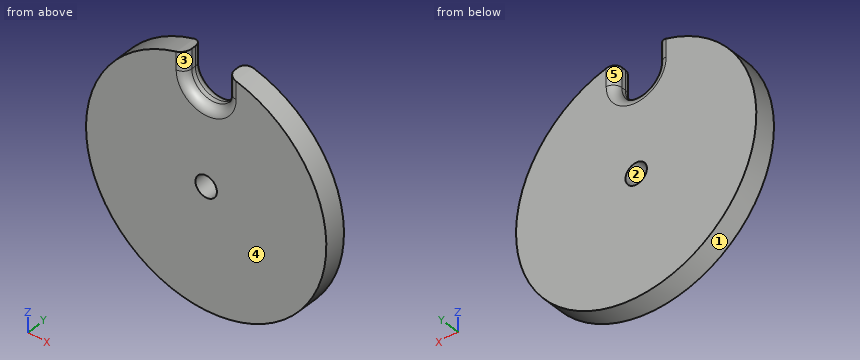
from build123d import *

# Parameters (mm, degrees)
SKETCH2_R                  = 35.56
BOSS_EXTRUDE1_DEPTH        = 6.35
SHOCK_CORD_HOLE_DEPTH      = 1
SHOCK_CORD_HOLE_DEPTH_BACK = 7.35
FILLET1_R                  = 2.54
SKETCH18_R                 = 3.175
CUT_EXTRUDE1_DEPTH         = 7.3500001


with BuildPart() as part:
    # Sketch2 → Boss-Extrude1 (new body)
    with BuildSketch(Plane(origin=(0, 0, 0), x_dir=(1, 0, 0), z_dir=(0, 1, 0))):
        Circle(SKETCH2_R)
    extrude(amount=BOSS_EXTRUDE1_DEPTH)

    # Sketch4 → Shock Cord hole (cut, two sides)
    with BuildSketch(Plane(origin=(0, 6.35, 0), x_dir=(1, 0, 0), z_dir=(0, 1, 0))) as shock_cord_hole_sk:
        with BuildLine():
            Line((6.35, -209.104630755), (6.35, -34.988442377))
            Line((6.35, -34.988442377), (6.35, -29.21))
            ThreePointArc((6.35, -29.21), (0, -22.86), (-6.35, -29.21))
            Line((-6.35, -29.21), (-6.35, -34.988442377))
            Line((-6.35, -34.988442377), (-6.35, -209.104630755))
            Line((-6.35, -209.104630755), (-6.35, -557.33700751))
            Line((-6.35, -557.33700751), (6.35, -557.33700751))
            Line((6.35, -557.33700751), (6.35, -209.104630755))
        make_face()
    extrude(amount=SHOCK_CORD_HOLE_DEPTH, mode=Mode.SUBTRACT)
    extrude(shock_cord_hole_sk.sketch, amount=-SHOCK_CORD_HOLE_DEPTH_BACK, mode=Mode.SUBTRACT)

    # Fillet1
    fillet1_edges = [part.edges().sort_by_distance(p)[0] for p in [
        (-6.35, 6.35, 32.099221189),
        (0, 6.35, 22.86),
        (6.35, 6.35, 32.099221189),
        (6.35, 0, 32.099221189),
        (0, 0, 22.86),
        (-6.35, 0, 32.099221189),
    ]]
    fillet(fillet1_edges, radius=FILLET1_R)

    # Sketch18 → Cut-Extrude1 (cut, through all)
    with BuildSketch(Plane.XZ):
        Circle(SKETCH18_R)
    extrude(amount=-CUT_EXTRUDE1_DEPTH, mode=Mode.SUBTRACT)


solid = part.part
Input: part model. Units: mm. Frame: model coordinates. Face numbers are marked on the shaded views. A direction names the side the tool comes from. Round coordinates to 2 decimals unless told otherwise and drop trailing zeros. Order: outer loops, then holes, each group sorted by start corner. A loop starts at its lowest first (then second) coordinate and runs counter-clockwise, first axis right, second up. Notation, with made-up numbers: (79.5, 56) - (99.5, 56) arc R15 ccw to (99.5, 63) - close; hole circle Ø10 at (79.5, 16). An arc over 180 degrees is marked (long way). Use a Markdown table: item, result.
1. Material intervals for probe 1 along Z at (x, y) = (0, 3) (3 decimals); probe 2 along X at (y, z) = (2.25, 0.5); probe 3 along X at (y, z) = (2.5, -2.5), sorted ascending.
Evaluation:
| item | result |
|---|---|
| probe 1 | -35.56 to -3.175, 3.175 to 22.86 |
| probe 2 | -35.56 to -3.14, 3.14 to 35.56 |
| probe 3 | -35.47 to -1.96, 1.96 to 35.47 |
2. Section A-A on x = 0. Return the cut outline in (y, z) (3 decimals), then the cut area to 3 significant figures.
Evaluation:
| item | result |
|---|---|
| outline | (0, -35.56) - (6.35, -35.56) - (6.35, -3.175) - (0, -3.175) - close; (0, 3.175) - (6.35, 3.175) - (6.35, 20.32) arc R2.54 ccw to (3.81, 22.86) - (2.54, 22.86) arc R2.54 ccw to (0, 20.32) - close |
| area | 328 mm^2 |
3. Mould query, pull axis Z, two halves, no side actions, for the marked faces 1, 2 and 3. Classes: +Z half, -Z half, draft (parallel to the pull), parting line (faces both ways), or undercut.
Evaluation:
| item | result |
|---|---|
| face 1 | parting line |
| face 2 | undercut |
| face 3 | draft |
4. Section D-D on z = -26.5. Return the cut outline in (x, y), then the cut area to 3 significant figures.
Evaluation:
| item | result |
|---|---|
| outline | (-23.71, 0) - (23.71, 0) - (23.71, 6.35) - (-23.71, 6.35) - close |
| area | 301 mm^2 |
5. Section C-C on y = 1.5. Return the cut outline in (x, z) (3 decimals).
Evaluation:
| item | result |
|---|---|
| outline | (-6.573, 29.21) - (-6.573, 34.947) arc R35.56 ccw (long way) to (6.573, 34.947) - (6.573, 29.21) arc R6.573 cw to start; hole circle Ø6.35 at (0, 0) |
6. Section B-B on z = 0. Return the cut outline in (x, y) (3 decimals).
Evaluation:
| item | result |
|---|---|
| outline | (-35.56, 0) - (-3.175, 0) - (-3.175, 6.35) - (-35.56, 6.35) - close; (3.175, 0) - (35.56, 0) - (35.56, 6.35) - (3.175, 6.35) - close |
7. Access query for the marked faces 4 and 5. Directions: +Z, -Z, +X, -X, +Y, -Y. A direction counts if a zero-diameter tool reaches every point of the face in a straight line with its end or side. Return the directions, or none.
Evaluation:
| item | result |
|---|---|
| face 4 | +Z, -Z, +X, -X, -Y |
| face 5 | +Z, +Y |
8. First-contact query: pin 1 (1 mm diameter, centred on x = -14, y = 2, fed in from -Z); pin 2 (1 mm diameter, centred on y = 3.5, z = 33.5, fed in from -X); pin 3 (3 mm diameter, centred on x = 15, y = 2, fed in from +Z). Flat tips, straight axial feed; report the tip coordinate or a pass-through.
Evaluation:
| item | result |
|---|---|
| pin 1 | z = -32.9 |
| pin 2 | x = -13.25 |
| pin 3 | z = 32.9 |
